```python
from build123d import *

# Parameters (mm, degrees)
F0_R     = 3.175
F1_DEPTH = 38.1
F3_DEPTH = 3.175
F4_R     = 1.5875
F5_DEPTH = 25.4


with BuildPart() as f1:
    # F0 (on Top) → F1 (new body)
    with BuildSketch(Plane.XY):
        Circle(F0_R)
    extrude(amount=F1_DEPTH)

    # F2 (on face) → F3 (join)
    with BuildSketch(Plane.XY.offset(38.1)):
        with BuildLine():
            Line((0, 3.175), (0.188579, 3.169395))
            ThreePointArc((0.188579, 3.169395), (0.094331, 3.173598), (0, 3.175))
        make_face()
        with BuildLine():
            Line((56.325018, 1.500813), (0.188579, 3.169395))
            Line((0.188579, 3.169395), (0, 3.175))
            ThreePointArc((0, 3.175), (-3.175, 0), (0, -3.175))
            Line((0, -3.175), (0.169236, -3.170486))
            Line((0.169236, -3.170486), (56.320177, -1.672922))
            ThreePointArc((56.320177, -1.672922), (57.865351, -0.088408), (56.325018, 1.500813))
        make_face()
        with BuildLine():
            Line((0.169236, -3.170486), (0, -3.175))
            ThreePointArc((0, -3.175), (0.084648, -3.173871), (0.169236, -3.170486))
        make_face()
    extrude(amount=F3_DEPTH)

    # F4 (on face) → F5 (join)
    with BuildSketch(Plane(origin=(0, 0, 38.1), x_dir=(1, 0, 0), z_dir=(0, 0, -1))):
        with Locations((56.277853, 0.085986)):
            Circle(F4_R)
    extrude(amount=F5_DEPTH)


solid = f1.part
```
The listing builds one solid part. Answer for the finished solid, in the listing's coordinates (mm). A direction names the side the tool comes from. Give positions to 0.01 mm unless a question says otherwise; leave off trailing zeros. Loops run counter-clockwise (first coordinate to the right, second up) from the corner with the lowest first, then second, coordinate; pieces in that order, holes last. Notation, with made-up numbers: (-5, 83.5) - (11, 83.5) arc R5 cw to (11, 92.5) - close; hole circle Ø10 at (22, -4). An arc over 180 degrees is marked (long way). Return JSON: item names as keys, results as strings. Group by question number.
1. Find section B-B (x = 2). Write down the section's boundary in (y, z) (3 decimals).
2. Straight lines are drawn through the part: line 1 (X direction, y = -0.25, z = 32); line 2 (X direction, y = -1.5, z = 24); line 3 (Z direction, x = 27, y = 0.5) (3 decimals). For each, find the intervals that lie inside material, in ascending order. Write a range as [from, to].
3. Determine the mould class of faces 3 (the flat face through (56, 0, 12.7)), 4 (the flat face through (28, 0, 38.1)) for opening direction X: pulls with the +X half, pulls with the -X half, needs draft (parallel to the pull), parting line crosses it, or undercut.
4. Given pin 1 Ø3.5 at (x, y) = (55.5, 0) entering from -Z; pin 2 Ø2 at (x, y) = (35, -2) entering from -Z, each flat-ended and moving along its own axis, determine where each tip first touches the part or whether it passes through.
5. Find section A-A (y = -0.75). Write down the section's boundary in (x, z) (3 decimals).
6. Find section D-D (z = 6). Write down the section's boundary in (x, y) (3 decimals).
7. Which of the six approach directions +Z, -Z, +X, -X, +Y, -Y give full straight-line access (tool end or side, diameter ignored) to faces 1 (the flat face through (0, 0, 0)), 2 (the cylindrical face through (-3.17, 0.14, 20.35))?
Verdict:
{
 "1": {"outline": "(-3.122, 38.1) - (-2.466, 38.1) - (-2.466, 0) - (2.466, 0) - (2.466, 38.1) - (3.116, 38.1) - (3.116, 41.275) - (-3.122, 41.275) - close"},
 "2": {"line 1": "x = [-3.17, 3.17], [54.7, 57.86]", "line 2": "x = [-2.8, 2.8], [55.56, 57]", "line 3": "z = [38.1, 41.275]"},
 "3": {"face 3": "needs draft", "face 4": "undercut"},
 "4": {"pin 1": "stops at z = 12.7", "pin 2": "stops at z = 38.1"},
 "5": {"outline": "(-3.085, 0) - (3.085, 0) - (3.085, 38.1) - (54.836, 38.1) - (54.836, 12.7) - (57.72, 12.7) - (57.72, 41.275) - (-3.085, 41.275) - close"},
 "6": {"outline": "circle Ø6.35 at (0, 0)"},
 "7": {"face 1": "-Z, +X, -X, +Y, -Y", "face 2": "-Z"}
}
